Autodesk Inventor part; units mm, degrees
ref_plane "YZ Plane" through (0, 0, 0) normal (1, 0, 0) x (0, 1, 0)
ref_plane "XZ Plane" through (0, 0, 0) normal (0, 1, 0) x (-1, 0, 0)
ref_plane "XY Plane" through (0, 0, 0) normal (0, 0, 1) x (1, 0, 0)
sketch "Sketch1" plane through (0, 0, 0) normal (0, 1, 0) x (-1, 0, 0)
  line L0 (0, 0) -> (19.4, 0)
  line L1 (19.4, 0) -> (19.4, -19.4)
  line L2 (19.4, -19.4) -> (0, -19.4)
  line L3 (0, -19.4) -> (0, 0)
  dimension "d0" = 19.4
  dimension "d1" = 19.4
extrude "Extrusion1" add sketch "Sketch1" along normal blind 4.5
sketch "Sketch2" plane through (0, 4.5, 0) normal (0, 1, 0) x (1, 0, 0)
  circle A0 centre (-3.6, 3.6) radius 1.6
  line L0 (-19.4, 0) -> (0, 0)
  line L1 (0, 0) -> (0, 19.4)
  dimension "d4" = 3.2
  dimension "d5" = 3.6
  dimension "d6" = 3.6
extrude "Extrusion2" cut sketch "Sketch2" against normal through all
pattern_linear "Rectangular Pattern1" count 2 spacing 12.2 along (0, 0, -1) count 2 spacing 12.2 along (-1, 0, 0) of "Extrusion2"
sketch "Sketch3" plane through (0, 0, 0) normal (1, 0, 0) x (0, 0, -1)
  line L0 (0.6, 2.5) -> (6.6, 2.5)
  line L1 (6.6, 2.5) -> (6.6, 0)
  line L2 (6.6, 0) -> (0.6, 0)
  line L3 (0.6, 0) -> (0.6, 2.5)
  line L4 (0, 0) -> (0, 4.5)
  line L5 (0, 0) -> (19.4, 0)
  line L6 (12.8, 2.5) -> (18.8, 2.5)
  line L7 (18.8, 2.5) -> (18.8, 0)
  line L8 (18.8, 0) -> (12.8, 0)
  line L9 (12.8, 0) -> (12.8, 2.5)
  line L10 (19.4, 0) -> (19.4, 4.5)
  dimension "d15" = 6
  dimension "d16" = 2.5
  dimension "d17" = 0.6
  dimension "d18" = 6
  dimension "d19" = 2.5
  dimension "d20" = 0.6
extrude "Extrusion3" cut sketch "Sketch3" against normal through all
properties part number "INTERFACE_MANIFOLD_KORK"
The listing builds one solid part. Answer for the finished solid, in the listing's coordinates (mm). A direction names the side the tool comes from. Round coordinates to 2 decimals unless told otherwise and drop trailing zeros. Write each loop counter-clockwise with the first axis right and the second up, starting at its lowest first coordinate (ties: lowest second). Pieces come first, ordered by that corner, then holes. Notation, with made-up numbers: (-25, 35) - (-3, 35) arc R22 ccw to (-3, 64) - close; hole circle Ø8 at (50, 79). An arc over 180 degrees is marked (long way). Use one line per item in the form item = value. Start each with the question number.
Item 1: Flat-ended cylindrical pins translate along their axes: pin 1 Ø5 at (x, z) = (-3.6, -15.8) entering from -Y; pin 2 Ø10 at (x, z) = (-12.5, -13.5) entering from -Y. Find the tip coordinate at first contact, or state that the pin passes through.
Item 2: Find the intervals of material crossed by line 1 (Z direction, x = -15.8, y = 3.3); line 2 (Z direction, x = -6, y = 2.05), in increasing order. Write a range as [from, to].
Item 3: A cutting plane is placed at D-D (x = -11.75). Write down the section's boundary in (y, z).
Item 4: Determine the mould class of faces 1 (the flat face through (-10, 1, -18.8)), 2 (the flat face through (-10, 2, -19.4)), 3 (the flat face through (-10, 0, -10)) for opening direction Z: +Z half, -Z half, draft (parallel to the pull), parting line (faces both ways), or undercut.
Item 5: A cutting plane is placed at B-B (x = -15.8). Write down the section's boundary in (y, z).
Item 6: A cutting plane is placed at C-C (z = -3.6). Write down the section's boundary in (x, y).
Item 7: A cutting plane is placed at A-A (y = 1.35). Write down the section's boundary in (x, z).
Item 8: A tool of negligible diameter and unlimited length cuts with its end or side. For faces 4 (the flat face through (-10, 2.5, -16)), 5 (the flat face through (0, 3, -10)), from which of +Z, -Z, +X, -X, +Y, -Y can it reach the whole face along a straight path? Write none if from no direction.
The answers:
q1.pin_1 = 2.5
q1.pin_2 = 0
q2.line_1 = [-19.4, -17.4], [-14.2, -5.2], [-2, 0]
q2.line_2 = [-19.4, -18.8], [-12.8, -6.6], [-0.6, 0]
q3.outline = (0, -19.4) - (4.5, -19.4) - (4.5, 0) - (0, 0) - (0, -0.6) - (2.5, -0.6) - (2.5, -6.6) - (0, -6.6) - (0, -12.8) - (2.5, -12.8) - (2.5, -18.8) - (0, -18.8) - close
q4.face_1 = undercut
q4.face_2 = -Z half
q4.face_3 = draft
q5.outline = (0, -19.4) - (4.5, -19.4) - (4.5, -17.4) - (2.5, -17.4) - (2.5, -18.8) - (0, -18.8) - close; (0, -12.8) - (2.5, -12.8) - (2.5, -14.2) - (4.5, -14.2) - (4.5, -5.2) - (2.5, -5.2) - (2.5, -6.6) - (0, -6.6) - close; (0, -0.6) - (2.5, -0.6) - (2.5, -2) - (4.5, -2) - (4.5, 0) - (0, 0) - close
q6.outline = (-19.4, 2.5) - (-17.4, 2.5) - (-17.4, 4.5) - (-19.4, 4.5) - close; (-14.2, 2.5) - (-5.2, 2.5) - (-5.2, 4.5) - (-14.2, 4.5) - close; (-2, 2.5) - (0, 2.5) - (0, 4.5) - (-2, 4.5) - close
q7.outline = (-19.4, -19.4) - (0, -19.4) - (0, -18.8) - (-19.4, -18.8) - close; (-19.4, -12.8) - (0, -12.8) - (0, -6.6) - (-19.4, -6.6) - close; (-19.4, -0.6) - (0, -0.6) - (0, 0) - (-19.4, 0) - close
q8.face_4 = +X, -X, -Y
q8.face_5 = +Z, -Z, +X, +Y, -Y
